Verification items for the finished model (mm, model axes). Face numbers are marked on the shaded views. Coordinates: 2 decimals unless noted, no trailing zeros. Loops run counter-clockwise (first coordinate to the right, second up) from the corner with the lowest first, then second, coordinate; pieces in that order, holes last. Notation, with made-up numbers: (-22, 87) -> (16, 87) arc R20 cw to (16, 98) -> close; hole circle Ø4 at (7.5, 55.5). An arc over 180 degrees is marked (long way). Write item = value, one per line.
```python
from build123d import *

# Parameters (mm, degrees)
F0_R     = 33
F0_R_2   = 30
F1_DEPTH = 92
F2_DEPTH = 3
F3_T     = -2.5
F4_R     = 1
F5_DEPTH = 6


with BuildPart() as f1:
    # F0 (on Front) → F1 (new body)
    with BuildSketch(Plane.XZ):
        Circle(F0_R)
        Circle(F0_R_2, mode=Mode.SUBTRACT)
        Circle(F0_R_2)
    extrude(amount=F1_DEPTH)

    # F0 (on Front) → F2 (join)
    with BuildSketch(Plane.XZ):
        Circle(F0_R)
        Circle(F0_R_2, mode=Mode.SUBTRACT)
    extrude(amount=F2_DEPTH)

    # F3
    f3_openings = [f1.faces().sort_by_distance(p)[0] for p in [
        (0, 0, 0),
    ]]
    offset(amount=F3_T, openings=f3_openings)

    # F4 (on face) → F5 (cut)
    with BuildSketch(Plane.XZ.offset(92)):
        with Locations((0, -28.224484995)):
            Circle(F4_R)
        with Locations((23.5754325986, 14.9141801521)):
            Circle(F4_R)
        with Locations((-22.5217076706, 16.2781162705)):
            Circle(F4_R)
    extrude(amount=-F5_DEPTH, mode=Mode.SUBTRACT)


solid = f1.part
```
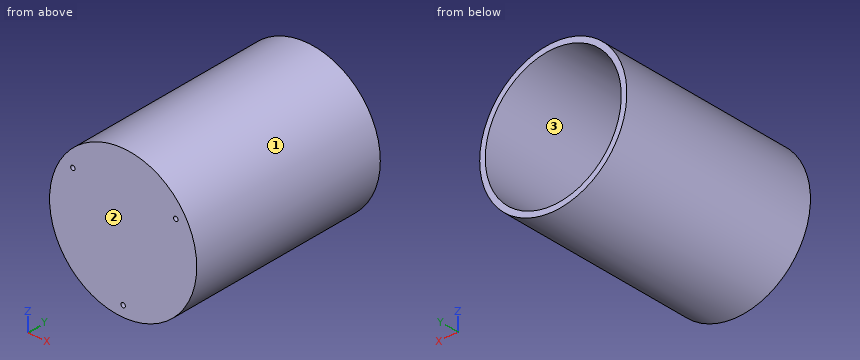
1) Release check for a two-part mould opening along X. For the marked faces 1, 2 and 3 record: pulls with the +X half, pulls with the -X half, needs draft (parallel to the pull), parting line crosses it, or undercut.
Ans:
face_1 = parting line crosses it
face_2 = needs draft
face_3 = undercut
2) Sectioned sample at B-B, the plane x = 3.5. Record the cut outline in (y, z), plus the area to 3 significant figures.
Ans:
outline = (-92, -32.81) -> (0, -32.81) -> (0, -30.3) -> (-89.5, -30.3) -> (-89.5, 30.3) -> (0, 30.3) -> (0, 32.81) -> (-92, 32.81) -> close
area = 614 mm2
3) Material ranges on line 1 (Z direction, x = 0, y = -90); line 2 (X direction, y = -26.5, z = 1); line 3 (Y direction, x = -22, z = 2), recorded low to high.
Ans:
line_1 = -33 to -29.22, -27.22 to 33
line_2 = -32.98 to -30.48, 30.48 to 32.98
line_3 = -92 to -89.5
4) Depth check by flat-ended pin: pin 1 Ø1.5 at (x, y) = (-3, -26) entering from -Z; pin 2 Ø1 at (x, z) = (24.5, 3) entering from +Y; pin 3 Ø10 at (x, y) = (-20.5, -55) entering from -Z; pin 4 Ø1.2 at (x, z) = (-22.52, 16.28) entering from -Y. Enter the tip coordinate at first touch or a pass-through.
Ans:
pin_1 = -32.92
pin_2 = -89.5
pin_3 = -29.13
pin_4 = through
5) Sectioned sample at C-C, the plane y = -78. Record the cut outline in (x, z).
Ans:
outline = circle Ø66 at (0, 0); hole circle Ø61 at (0, 0)
6) Sectioned sample at A-A, the plane z = 0. Record the cut outline in (x, y).
Ans:
outline = (-33, -92) -> (33, -92) -> (33, 0) -> (30.5, 0) -> (30.5, -89.5) -> (-30.5, -89.5) -> (-30.5, 0) -> (-33, 0) -> close
